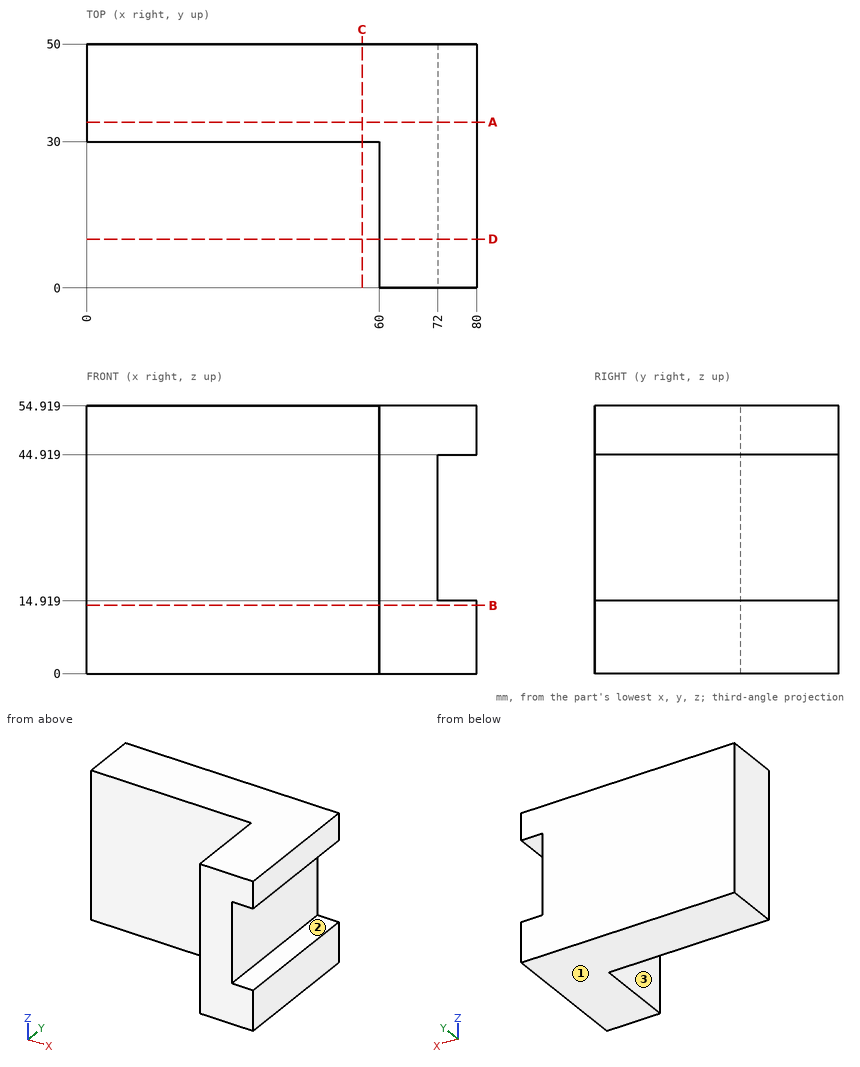
Study the drawing (mm; zero at the part's minimum x, y, z) and answer. A direction names the side the tool comes from. Give positions to 0.01 mm unless a question says otherwise; leave off trailing zeros. Loops run counter-clockwise (first coordinate to the right, second up) from the corner with the lowest first, then second, coordinate; pieces in that order, holes last. Notation, with made-up numbers: (-25.75, 22.5) - (22.25, 22.5) arc R24 cw to (22.25, 43.5) - close; hole circle Ø1 at (-38, -25). An arc over 180 degrees is marked (long way). Use CSV: the item, a comma, the result in double quotes. Start each with the question number.
(1) A tool of negligible diameter and unlimited length cuts with its end or side. For the marked faces 1, 2 and 3, from which of +Z, -Z, +X, -X, +Y, -Y can it reach the whole face along a straight path? Write none if from no direction.
(2) Find section C-C, the plane x = 56.5. Determine the outline of the cut face in (y, z), plus the area to 3 significant figures.
(3) Each of these flat-tipped pins is pushed along its axis until it touches: pin 1 (15 mm diameter, centred on y = 21, z = 39, fed in from -X); pin 2 (1 mm diameter, centred on y = 22, z = 36.5, fed in from +X); pin 3 (4 mm diameter, centred on x = 9, z = 47, fed in from -Y). Where does it stop, or does it pass through?
(4) Find section B-B, the plane z = 14. Determine the outline of the cut face in (x, y).
(5) Find the intervals of material crossed by L1, parallel to Z at x = 75, y = 11; L2, parallel to X at y = 10.5, z = 3; L3, parallel to X at y = 6, z = 16, in increasing order.
(6) Find section D-D, the plane y = 10. Determine the outline of the cut face in (x, z), plus the area to 3 significant figures.
(7) Find section A-A, the plane y = 34. Determine the outline of the cut face in (x, z), plus the area to 3 significant figures.
Results found:
1,face 1,"-Z, +X, -X, +Y, -Y"
1,face 2,"+X, +Y, -Y"
1,face 3,"+Z, -Z, -X, -Y"
2,outline,"(30, 0) - (50, 0) - (50, 54.92) - (30, 54.92) - close"
2,area,"1,100 mm^2"
3,pin 1,"x = 60"
3,pin 2,"x = 72"
3,pin 3,"y = 30"
4,outline,"(0, 30) - (60, 30) - (60, 0) - (80, 0) - (80, 50) - (0, 50) - close"
5,L1,"0 to 14.92, 44.92 to 54.92"
5,L2,"60 to 80"
5,L3,"60 to 72"
6,outline,"(60, 0) - (80, 0) - (80, 14.92) - (72, 14.92) - (72, 44.92) - (80, 44.92) - (80, 54.92) - (60, 54.92) - close"
6,area,"858 mm^2"
7,outline,"(0, 0) - (80, 0) - (80, 14.92) - (72, 14.92) - (72, 44.92) - (80, 44.92) - (80, 54.92) - (0, 54.92) - close"
7,area,"4,150 mm^2"
